```python
from build123d import *

# Parameters (mm, degrees)
SKETCH1_W           = 60
SKETCH1_H           = 30
BOSS_EXTRUDE1_DEPTH = 5
SKETCH2_W           = 10
SKETCH2_H           = 5
CUT_EXTRUDE1_DEPTH  = 10
FILLET1_R           = 0.5


with BuildPart() as part:
    # Sketch1 → Boss-Extrude1 (new body)
    with BuildSketch(Plane(origin=(0, 0, 0), x_dir=(1, 0, 0), z_dir=(0, 1, 0))):
        with Locations((-486.052613816, 355.540919523)):
            Rectangle(SKETCH1_W, SKETCH1_H)
    extrude(amount=BOSS_EXTRUDE1_DEPTH)

    # Sketch2 → Cut-Extrude1 (cut)
    with BuildSketch(Plane(origin=(0, 0, -370.540919523), x_dir=(-1, 0, 0), z_dir=(0, 0, -1))):
        with Locations((486.052613816, 2.5)):
            Rectangle(SKETCH2_W, SKETCH2_H)
    extrude(amount=-CUT_EXTRUDE1_DEPTH, mode=Mode.SUBTRACT)

    # Fillet1
    fillet1_edges = [part.edges().sort_by_distance(p)[0] for p in [
        (-456.052613816, 5, -355.540919523),
        (-503.552613816, 5, -370.540919523),
        (-468.552613816, 0, -370.540919523),
        (-468.552613816, 5, -370.540919523),
        (-481.052613816, 5, -365.540919523),
        (-491.052613816, 2.5, -370.540919523),
        (-491.052613816, 5, -365.540919523),
        (-486.052613816, 0, -360.540919523),
        (-491.052613816, 0, -365.540919523),
        (-481.052613816, 2.5, -360.540919523),
        (-481.052613816, 0, -365.540919523),
        (-486.052613816, 5, -360.540919523),
        (-491.052613816, 2.5, -360.540919523),
        (-481.052613816, 2.5, -370.540919523),
        (-516.052613816, 5, -355.540919523),
        (-503.552613816, 0, -370.540919523),
        (-486.052613816, 5, -340.540919523),
        (-516.052613816, 2.5, -370.540919523),
        (-456.052613816, 2.5, -370.540919523),
    ]]
    fillet(fillet1_edges, radius=FILLET1_R)


solid = part.part
```
Read the model definition and answer for the solid it produces. Units are mm, in the model's axes. A direction names the side the tool comes from. Coordinates: 2 decimals unless noted, no trailing zeros. Order: outer loops, then holes, each group sorted by start corner. A loop starts at its lowest first (then second) coordinate and runs counter-clockwise, first axis right, second up. Notation, with made-up numbers: (14.25, 73) - (22.25, 73) arc R34 cw to (22.25, 112) - close; hole circle Ø9 at (32, 12.5). An arc over 180 degrees is marked (long way). Answer as a JSON object with one key per item and string values. Group by question number.
Item 1: Section C-C (y = 2.15) is taken. Give the vertices of the cut face in (x, z).
Item 2: Consider probe 1 along X at (y, z) = (2.7, -368.5); probe 2 along Z at (x, y) = (-466, 4.6); probe 3 along X at (y, z) = (4.85, -361.75). Determine where each line is inside the solid, lowest interval first. Write a range as from..to.
Item 3: The mould has two halves that part along X. Classify faces 1 (the face through (-456.053, 2, -355)), 2 (the face through (-516.053, 2, -355)), 3 (the face through (-481.053, 2, -366)), 4 (the face through (-486, 2, -340.541)): +X half, -X half, draft (parallel to the pull), parting line (faces both ways), or undercut.
Item 4: Section A-A (z = -367.5) is taken. Give the vertices of the cut face in (x, y).
Item 5: A tool of negligible diameter and unlimited length cuts with its end or side. For faces 5 (the face through (-486, 5, -356)), 6 (the face through (-491.053, 2, -366)), from which of +Z, -Z, +X, -X, +Y, -Y can it reach the whole face along a straight path? Write none if from no direction.
Item 6: A flat-ended cylindrical pin translates along its axis: P1, Ø3, axis at x = -484, y = 2, coming from the -Z side. Find the tip coordinate at first contact, or state that the pin passes through.
Item 7: Section B-B (x = -489) is taken. Give the vertices of the cut face in (y, z).
Results are:
{
 "1": {"outline": "(-516.05, -370.04) arc R0.5 ccw to (-515.55, -370.54) - (-491.55, -370.54) arc R0.5 ccw to (-491.05, -370.04) - (-491.05, -361.04) arc R0.5 cw to (-490.55, -360.54) - (-481.55, -360.54) arc R0.5 cw to (-481.05, -361.04) - (-481.05, -370.04) arc R0.5 ccw to (-480.55, -370.54) - (-456.55, -370.54) arc R0.5 ccw to (-456.05, -370.04) - (-456.05, -340.54) - (-516.05, -340.54) - close"},
 "2": {"probe 1": "x = -516.05..-491.05, -481.05..-456.05", "probe 2": "z = -370.53..-340.55", "probe 3": "x = -515.91..-491.2, -480.91..-456.2"},
 "3": {"face 1": "+X half", "face 2": "-X half", "face 3": "undercut", "face 4": "draft"},
 "4": {"outline": "(-516.05, 0) - (-491.55, 0) arc R0.5 ccw to (-491.05, 0.5) - (-491.05, 4.5) arc R0.5 ccw to (-491.55, 5) - (-515.55, 5) arc R0.5 ccw to (-516.05, 4.5) - close; (-481.05, 0.5) arc R0.5 ccw to (-480.55, 0) - (-456.05, 0) - (-456.05, 4.5) arc R0.5 ccw to (-456.55, 5) - (-480.55, 5) arc R0.5 ccw to (-481.05, 4.5) - close"},
 "5": {"face 5": "+Z, -Z, +X, -X, +Y", "face 6": "-Z, +Y, -Y"},
 "6": {"P1": "stops at z = -360.54"},
 "7": {"outline": "(0, -360.04) arc R0.5 ccw to (0.5, -360.54) - (4.5, -360.54) arc R0.5 ccw to (5, -360.04) - (5, -341.04) arc R0.5 ccw to (4.5, -340.54) - (0, -340.54) - close"}
}
